Autodesk Inventor part; units mm, degrees
ref_plane "YZ Plane" through (0, 0, 0) normal (1, 0, 0) x (0, 1, 0)
ref_plane "XZ Plane" through (0, 0, 0) normal (0, 1, 0) x (-1, 0, 0)
ref_plane "XY Plane" through (0, 0, 0) normal (0, 0, 1) x (1, 0, 0)
sketch "Sketch4" plane through (0, 0, 0) normal (1, 0, 0) x (0, 1, 0)
  line L0 (0, 0) -> (0, -12.7)
  line L1 (0, -12.7) -> (-101.6, 0)
  line L2 (-101.6, 0) -> (-101.6, -12.7)
  line L3 (-101.6, -12.7) -> (-203.2, 0)
  line L4 (-203.2, 0) -> (-203.2, -12.7)
  line L5 (-203.2, -12.7) -> (-304.8, 0)
  line L6 (-82.55, -2.3812) -> (-82.55, 7.7787)
  line L7 (-82.55, 7.7787) -> (-234.95, 7.7787)
  line L8 (-234.95, 7.7787) -> (-234.95, -8.7313)
  dimension "d28" = 12.7
  dimension "d29" = 101.6
  dimension "d30" = 101.6
  dimension "d31" = 12.7
  dimension "d32" = 101.6
  dimension "d33" = 152.4
  dimension "d34" = 10.16
  dimension "d35" = 19.05
extrude "Extrusion3" add sketch "Sketch4" along normal mid plane 152.4
sketch "Sketch5" plane through (-76.2, -234.95, 7.7787) normal (0, 0, 1) x (1, 0, 0)
  line L0 (0, 0) -> (0, 152.4) construction
  line L1 (0, 152.4) -> (152.3647, 0) construction
  line L2 (152.4, 152.4) -> (152.4, 0) construction
  line L3 (0, 0) -> (152.4, 0) construction
  line L4 (152.4, 152.4) -> (0, 0) construction
  line L5 (6.35, 6.35) -> (146.05, 6.35) construction
  line L6 (146.05, 6.35) -> (146.05, 146.05) construction
  line L7 (146.05, 146.05) -> (6.35, 146.05) construction
  line L8 (6.35, 146.05) -> (6.35, 6.35) construction
  line L9 (6.35, 6.35) -> (146.05, 146.05) construction
  line L10 (146.05, 6.35) -> (6.35, 146.05) construction
  line L11 (0, 152.4) -> (152.4, 152.4) construction
  circle A0 centre (76.2, 76.2) radius 57.15
  line L12 (76.2, 19.05) -> (76.2, 0) construction
  line L13 (0, 0) -> (152.4, 0) construction
  line L14 (76.454, 0) -> (76.454, 19.0506)
  line L15 (75.946, 0) -> (75.946, 19.0506)
  line L16 (75.946, 0) -> (76.454, 0)
  point P0 (76.2, 234.95)
  point P1 (75.946, 19.0506)
  dimension "d38" = 6.35
  dimension "d39" = 6.35
  dimension "d40" = 114.3
  dimension "d51" = 0.254
extrude "Extrusion4" cut sketch "Sketch5" against normal through all contours A0
hole "Hole2" at (-69.85, -88.9, 7.7787) at (69.85, -88.9, 7.7787) at (69.85, -228.6, 7.7787) at (-69.85, -228.6, 7.7787) direction (0, 0, -1) diameter 6.7564 end through all
fillet "Fillet2" radius 6.35 4 edges at (76.2, -82.55, 2.6987) (-76.2, -82.55, 2.6987) (76.2, -234.95, -0.4763) (-76.2, -234.95, -0.4763)
extrude "Extrusion5" cut sketch "Sketch5" against normal through all contours A0 L14 L16 L15
fillet "Fillet3" radius 1.5875 2 edges at (40.5009, -199.0712, 7.7787) (-40.3212, -118.2491, 7.7787)
fillet "Fillet4" radius 1.5875 9 edges at (74.3401, -84.4099, 7.7787) (76.2, -158.75, 7.7787) (74.3401, -233.0901, 7.7787) (35.052, -234.95, 7.7787) (-74.3401, -84.4099, 7.7787) (-76.2, -158.75, 7.7787) (-74.3401, -233.0901, 7.7787) (-35.052, -234.95, 7.7787) (0, -82.55, 7.7787)
fillet "Fillet5" radius 1.5875 17 edges at (76.2, -152.4, -6.35) (-76.2, -152.4, -6.35) (-74.3401, -233.0901, -8.9637) (-35.052, -234.95, -8.7313) (-76.2, -215.9, -11.1125) (74.3401, -233.0901, -8.9637) (35.052, -234.95, -8.7313) (76.2, -215.9, -11.1125) (76.2, -203.2, -6.35) (-76.2, -203.2, -6.35) (-76.2, -101.6, -6.35) (76.2, -101.6, -6.35) (74.3401, -84.4099, -2.1488) (76.2, -95.25, -0.7937) (-74.3401, -84.4099, -2.1488) (-76.2, -95.25, -0.7937) (0, -82.55, -2.3812)
equation "\"d36\" = outsideWidthOfVent"
equation "\"d40\" = ventHole"
equation "\"d50\" = ventRadius"
equation "\"sidingHeight\" = 101.6"
equation "\"sidingDepth\" = 12.7"
equation "\"radiusOfCurvature\" = 609.6"
equation "\"outsideWidthOfVent\" = 152.4"
equation "\"wallThicknessOfVent\" = 19.05"
equation "\"holeOffset\" = 6.35"
equation "\"ventHole\" = 114.3"
equation "\"ventRadius\" = 6.35"
properties part number "ventForDryer02"
Here's how the part is built. I have some questions about the finished solid (model axes, mm). A direction names the side the tool comes from. Give positions to 0.01 mm unless a question says otherwise; leave off trailing zeros. Write each question's results on one line, items separated by ' | '.
Item 1: If I drill on L1, parallel to Y at x = -69.85, z = 5.5; L2, parallel to X at y = -88.9, z = 5.25; L3, parallel to X at y = -228.6, z = 2, over which ranges is the centre line in solid material (lowest first)?
Output:
L1: y = -234.95 to -231.98, -225.22 to -92.28, -85.52 to -82.55 | L2: x = -76.2 to -73.23, -66.47 to 66.47, 73.23 to 76.2 | L3: x = -76.2 to -73.23, -66.47 to -0.25, 0.25 to 66.47, 73.23 to 76.2
Item 2: For pin 1 Ø6.5 at (x, z) = (49, -5) entering from +Y; pin 2 Ø9 at (x, y) = (-69.85, -88.9) entering from -Z; pin 3 Ø10 at (y, z) = (-193.5, -5) entering from -X, each with a flat end and sliding along its axis, tell me the tip position at first contact or that it passes through.
Output:
pin 1: stops at y = -83.06 | pin 2: stops at z = -2.15 | pin 3: stops at x = -76.16
Item 3: On a 3-axis mill with a long thin cutter (end or side, diameter ignored), from which of +Z, -Z, +X, -X, +Y, -Y can I reach the whole of each face in a straight line? I mean faces 4 (the face through (-0.254, -226, -2)), 5 (the face through (-1, -92.8, -1.1)), 6 (the face through (-75.75, -96.28, -0.18)). Say none if no direction works.
Output:
face 4: +Z, -Z, -Y | face 5: -Z, +X, -X | face 6: -Z, -X
Item 4: We'd pull the mould along X, two halves only. Please class faces 1 (the face through (55, -203.2, -6)), 2 (the face through (-68.556, -231.721, -1.211)), 3 (the face through (75.747, -96.081, -0.209)): pulls with the +X half, pulls with the -X half, needs draft (parallel to the pull), parting line crosses it, or undercut.
Output:
face 1: needs draft | face 2: undercut | face 3: pulls with the +X half
